Design review of the part shown in the three views and the two pictorial views. Dimensions are in mm from the part's minimum x, y and z. A direction names the side the tool comes from. Coordinates: 2 decimals unless noted, no trailing zeros. Loops run counter-clockwise (first coordinate to the right, second up) from the corner with the lowest first, then second, coordinate; pieces in that order, holes last.
Q1. Draft analysis for pull direction Y (two halves, no side actions). For the marked faces 3, 4 and 5, state which applies: released by +Y, released by -Y, zero draft, split by the parting line, or undercut.
Q2. For P1, Ø5.5, axis at x = 7.5, z = 7.5, coming from the -Y side; P2, Ø6.5, axis at x = 8.5, z = 5, coming from the +Y side, all flat-tipped, find the tip position at first contact; note any pin that passes through.
Q3. Add section B-B on z = 7.5. Give the boundary of the cut face in (x, y).
Q4. Add section C-C on x = 3. Give the boundary of the cut face in (y, z), and give its area (3 significant figures).
Q5. Wall thickness on probe 1 along Z at (x, y) = (7.5, 14.6); probe 2 along Y at (x, z) = (12.25, 3): over which ranges is each line inside the solid? List them lowest first.
Q6. Machinability: for the marked faces 1 and 2, which of the approach directions +Z, -Z, +X, -X, +Y, -Y give a long, thin tool a straight path to every point of the face, cutting with its end or side? Answer none if there is none.
Q7. Add section A-A on y = 7.5. Give the boundary of the cut face in (x, z).
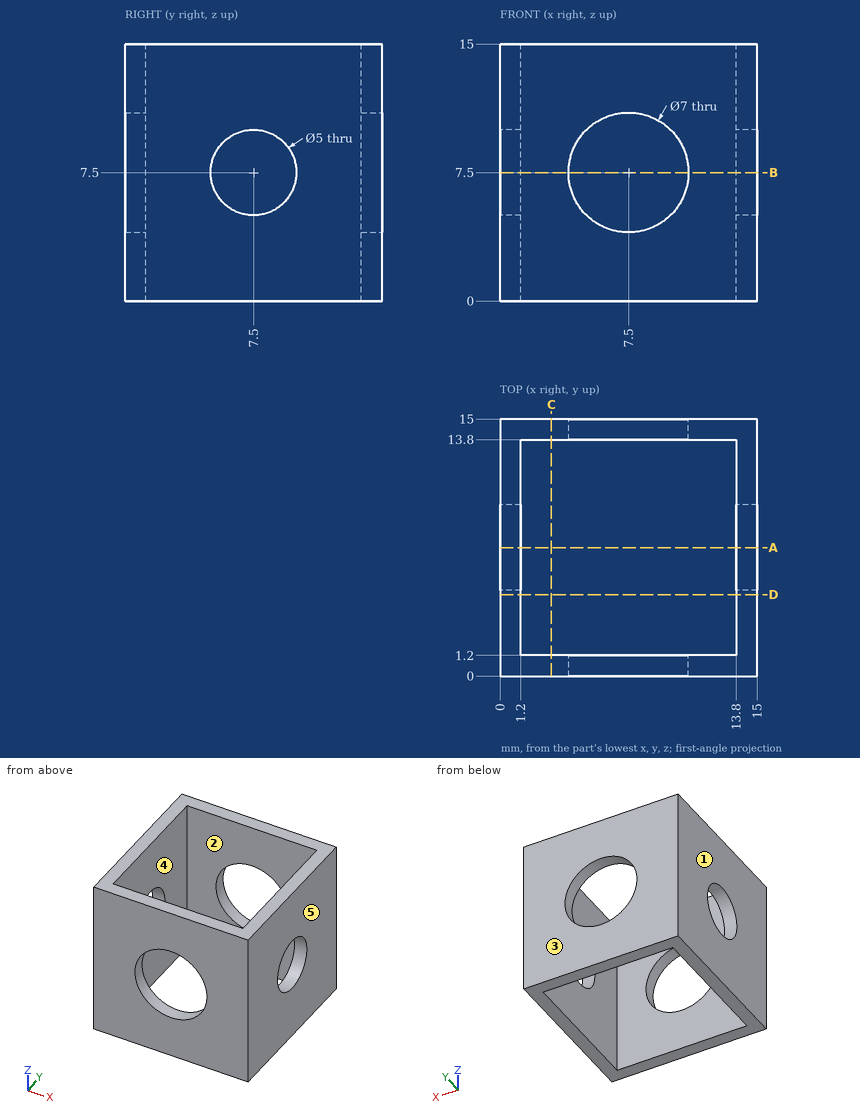
Entries:
1. face 3: released by +Y
1. face 4: undercut
1. face 5: zero draft
2. P1: passes through
2. P2: stops at y = 15
3. outline: (0, 0) - (4, 0) - (4, 1.2) - (1.2, 1.2) - (1.2, 5) - (0, 5) - close; (0, 10) - (1.2, 10) - (1.2, 13.8) - (4, 13.8) - (4, 15) - (0, 15) - close; (11, 0) - (15, 0) - (15, 5) - (13.8, 5) - (13.8, 1.2) - (11, 1.2) - close; (11, 13.8) - (13.8, 13.8) - (13.8, 10) - (15, 10) - (15, 15) - (11, 15) - close
4. outline: (0, 0) - (1.2, 0) - (1.2, 15) - (0, 15) - close; (13.8, 0) - (15, 0) - (15, 15) - (13.8, 15) - close
4. area: 36.0 mm2
5. probe 1: z = 0 to 4, 11 to 15
5. probe 2: y = 0 to 1.2, 13.8 to 15
6. face 1: +Z, -Z, -X, +Y, -Y
6. face 2: +Z, -Z
7. outline: (0, 0) - (1.2, 0) - (1.2, 5) - (0, 5) - close; (0, 10) - (1.2, 10) - (1.2, 15) - (0, 15) - close; (13.8, 0) - (15, 0) - (15, 5) - (13.8, 5) - close; (13.8, 10) - (15, 10) - (15, 15) - (13.8, 15) - close
